Model file for the job. Use its own axes, mm. A direction names the side the tool comes from. Give positions to 0.01 mm unless a question says otherwise; leave off trailing zeros. Write each loop counter-clockwise with the first axis right and the second up, starting at its lowest first coordinate (ties: lowest second). Pieces come first, ordered by that corner, then holes.
```python
from build123d import *

# Parameters (mm, degrees)
EXTRUDE_1_DEPTH      = 1.5
EXTRUDE_1_DEPTH_BACK = 3
SKETCH_1_W           = 5
SKETCH_1_H           = 5
SKETCH_3_W           = 16.55
SKETCH_3_H           = 2
EXTRUDE_2_DEPTH      = 1
SKETCH_4_W           = 2.010575614
SKETCH_4_H           = 1.682122854
EXTRUDE_3_DEPTH      = 1
SKETCH_5_W           = 2
SKETCH_5_H           = 1.650542366
EXTRUDE_4_DEPTH      = 1


with BuildPart() as part:
    # 草图1 → 凸台-拉伸1 (new, two sides: drawn at the far end of the back side and taken through both)
    with BuildSketch(Plane(origin=(0, 0, 0), x_dir=(1, 0, 0), z_dir=(0, 1, 0)).offset(-EXTRUDE_1_DEPTH_BACK)):
        Rectangle(SKETCH_1_W, SKETCH_1_H)
    extrude(amount=EXTRUDE_1_DEPTH + EXTRUDE_1_DEPTH_BACK)

    # 草图2 → 旋转1 (revolve)
    with BuildSketch(Plane.XY):
        with BuildLine():
            Line((-6, -6.817094506), (0, -6.817094506))
            Line((0, -6.817094506), (0, -1.613202234))
            add(Edge.make_bspline(
                [(-6, -6.817094506), (-4.734338842, -2.184392528), (0, -1.613202234)],
                knots=[0, 0, 0, 1, 1, 1], degree=2))
        make_face()
    revolve(axis=Axis((0, -6.817094506, 0), (0, 1, 0)))

    # 草图3 → 凸台-拉伸2 (add)
    with BuildSketch(Plane.XZ.offset(6.817094506)):
        Rectangle(SKETCH_3_W, SKETCH_3_H)
    extrude(amount=EXTRUDE_2_DEPTH)

    # 草图4 → 凸台-拉伸3 (add)
    with BuildSketch(Plane.ZY.offset(8.275)):
        with Locations((0.005287807, -6.976033079)):
            Rectangle(SKETCH_4_W, SKETCH_4_H)
    extrude(amount=EXTRUDE_3_DEPTH)

    # 草图5 → 凸台-拉伸4 (add)
    with BuildSketch(Plane(origin=(8.275, 0, 0), x_dir=(0, 0, -1), z_dir=(1, 0, 0))):
        with Locations((0, -6.991823323)):
            Rectangle(SKETCH_5_W, SKETCH_5_H)
    extrude(amount=EXTRUDE_4_DEPTH)


solid = part.part
```
1. Which spindle directions (+Z, -Z, +X, -X, +Y, -Y) get a long thin tool onto all of the face, cutting with end or side? Do faces 4 (the flat face through (-9, -6.135, 0)), 5 (the flat face through (0, -6.817, -3)), 6 (the flat face through (9, -6.167, 0)), 7 (the flat face through (-9, -7, 1.011)). Say none if no direction does.
Calculated:
face 4: +Z, -Z, -X, +Y
face 5: -Z, +X, -X, -Y
face 6: +Z, -Z, +X, +Y
face 7: +Z, -X, +Y, -Y
2. Slice it at B-B, the plane x = -8. Write the cut outline in (y, z).
Calculated:
outline: (-7.82, -1) - (-6.82, -1) - (-6.82, 1) - (-7.82, 1) - close
3. Slice it at A-A, the plane y = -0.25. Write the cut outline in (x, z).
Calculated:
outline: (-2.5, -2.5) - (2.5, -2.5) - (2.5, 2.5) - (-2.5, 2.5) - close
4. Pin check, flat tips, straight feed: P1, Ø3, axis at y = -2.5, z = -3.5, coming from the -X side; P2, Ø5, axis at y = -0.5, z = -0.5, coming from the +X side; P3, Ø1.3, axis at x = -1, y = -0.5, coming from the +Z side; P4, Ø5.5, axis at x = 1, z = 3.5, coming from the -Y side. Stop position of each tip, or through.
Calculated:
P1: stops at x = -3.53
P2: stops at x = 3.6
P3: stops at z = 2.5
P4: stops at y = -7.82
5. Probe probe 1 along X at (y, z) = (0.25, -1); probe 2 along Y at (x, z) = (2.75, -4.75); probe 3 along Y at (x, z) = (3.75, 1.5). List the from-to ranges inside material, lowest first.
Calculated:
probe 1: x = -2.5 to 2.5
probe 2: y = -6.82 to -5.4
probe 3: y = -6.82 to -3.35
6. Pull direction X, two halves, no side cores. Call faces 1 (the flat face through (9.275, -7, 0)), 2 (the flat face through (0, -7, 1)), 3 (the flat face through (7, -6.817, 0)): +X half, -X half, draft (parallel to the pull), parting line (faces both ways), or undercut.
Calculated:
face 1: +X half
face 2: draft
face 3: undercut
